from build123d import *

# Parameters (mm, degrees)
SKETCH2_R           = 6
SKETCH2_R_2         = 1.5
BOSS_EXTRUDE1_DEPTH = 1.15
SKETCH3_R           = 4.4
BOSS_EXTRUDE2_DEPTH = 3.2
SKETCH5_R           = 10
SKETCH5_R_2         = 0.75
SKETCH5_R_3         = 1.5
BOSS_EXTRUDE4_DEPTH = 1.15


with BuildPart() as part:
    # Sketch2 → Boss-Extrude1 (new body, symmetric)
    with BuildSketch(Plane(origin=(0, 0, 0), x_dir=(1, 0, 0), z_dir=(0, 1, 0))):
        Circle(SKETCH2_R)
        Circle(SKETCH2_R_2, mode=Mode.SUBTRACT)
    extrude(amount=BOSS_EXTRUDE1_DEPTH, both=True)

    # Sketch3 → Boss-Extrude2 (add)
    with BuildSketch(Plane(origin=(0, 1.15, 0), x_dir=(1, 0, 0), z_dir=(0, 1, 0))):
        Circle(SKETCH3_R)
        with BuildLine():
            Line((0.107421435, 2.898009771), (0.338399731, 2.678709694))
            Line((0.338399731, 2.678709694), (0.61665913, 2.83367809))
            ThreePointArc((0.61665913, 2.83367809), (0.721200673, 2.808891167), (0.824752316, 2.780248841))
            Line((0.824752316, 2.780248841), (0.993936292, 2.510396512))
            Line((0.993936292, 2.510396512), (1.301992734, 2.591295993))
            ThreePointArc((1.301992734, 2.591295993), (1.397085655, 2.541289372), (1.490260976, 2.48779465))
            Line((1.490260976, 2.48779465), (1.587020181, 2.184345885))
            Line((1.587020181, 2.184345885), (1.905517346, 2.186093238))
            ThreePointArc((1.905517346, 2.186093238), (1.985186607, 2.11400902), (2.062131058, 2.039023173))
            Line((2.062131058, 2.039023173), (2.080385755, 1.721044772))
            Line((2.080385755, 1.721044772), (2.389311295, 1.643530205))
            ThreePointArc((2.389311295, 1.643530205), (2.448550984, 1.553897705), (2.504429862, 1.46213237))
            Line((2.504429862, 1.46213237), (2.443033042, 1.149604087))
            Line((2.443033042, 1.149604087), (2.722976028, 0.997698125))
            ThreePointArc((2.722976028, 0.997698125), (2.758063897, 0.896149284), (2.789366126, 0.793370413))
            Line((2.789366126, 0.793370413), (2.652175577, 0.505929549))
            Line((2.652175577, 0.505929549), (2.885546163, 0.289177003))
            ThreePointArc((2.885546163, 0.289177003), (2.894277512, 0.182092507), (2.899036259, 0.074758075))
            Line((2.899036259, 0.074758075), (2.694672167, -0.169534403))
            Line((2.694672167, -0.169534403), (2.866806821, -0.437514174))
            ThreePointArc((2.866806821, -0.437514174), (2.848633027, -0.543405812), (2.826549281, -0.648551587))
            Line((2.826549281, -0.648551587), (2.567852594, -0.834345885))
            Line((2.567852594, -0.834345885), (2.667935462, -1.136714727))
            ThreePointArc((2.667935462, -1.136714727), (2.623998452, -1.234759946), (2.576459817, -1.331110368))
            Line((2.576459817, -1.331110368), (2.279685399, -1.446732346))
            Line((2.279685399, -1.446732346), (2.301427906, -1.764491312))
            ThreePointArc((2.301427906, -1.764491312), (2.234488404, -1.84852957), (2.164481907, -1.930030589))
            Line((2.164481907, -1.930030589), (1.848277186, -1.968215294))
            Line((1.848277186, -1.968215294), (1.790313171, -2.281398419))
            ThreePointArc((1.790313171, -2.281398419), (1.704577232, -2.346149284), (1.616501638, -2.40767989))
            Line((1.616501638, -2.40767989), (1.30073492, -2.366028036))
            Line((1.30073492, -2.366028036), (1.166706475, -2.654956874))
            ThreePointArc((1.166706475, -2.654956874), (1.067561203, -2.696351809), (0.966950626, -2.734045809))
            Line((0.966950626, -2.734045809), (0.671462695, -2.615174535))
            Line((0.671462695, -2.615174535), (0.469791321, -2.861694623))
            ThreePointArc((0.469791321, -2.861694623), (0.363466377, -2.877132634), (0.25664255, -2.888621575))
            Line((0.25664255, -2.888621575), (0, -2.7))
            Line((0, -2.7), (-0.25664255, -2.888621575))
            ThreePointArc((-0.25664255, -2.888621575), (-0.363466377, -2.877132634), (-0.469791321, -2.861694623))
            Line((-0.469791321, -2.861694623), (-0.671462695, -2.615174535))
            Line((-0.671462695, -2.615174535), (-0.966950626, -2.734045809))
            ThreePointArc((-0.966950626, -2.734045809), (-1.067561203, -2.696351809), (-1.166706475, -2.654956874))
            Line((-1.166706475, -2.654956874), (-1.30073492, -2.366028036))
            Line((-1.30073492, -2.366028036), (-1.616501638, -2.40767989))
            ThreePointArc((-1.616501638, -2.40767989), (-1.704577232, -2.346149284), (-1.790313171, -2.281398419))
            Line((-1.790313171, -2.281398419), (-1.848277186, -1.968215294))
            Line((-1.848277186, -1.968215294), (-2.164481907, -1.930030589))
            ThreePointArc((-2.164481907, -1.930030589), (-2.234488404, -1.84852957), (-2.301427906, -1.764491312))
            Line((-2.301427906, -1.764491312), (-2.279685399, -1.446732346))
            Line((-2.279685399, -1.446732346), (-2.576459817, -1.331110368))
            ThreePointArc((-2.576459817, -1.331110368), (-2.623998452, -1.234759946), (-2.667935462, -1.136714727))
            Line((-2.667935462, -1.136714727), (-2.567852594, -0.834345885))
            Line((-2.567852594, -0.834345885), (-2.826549281, -0.648551587))
            ThreePointArc((-2.826549281, -0.648551587), (-2.848633027, -0.543405812), (-2.866806821, -0.437514174))
            Line((-2.866806821, -0.437514174), (-2.694672167, -0.169534403))
            Line((-2.694672167, -0.169534403), (-2.899036259, 0.074758075))
            ThreePointArc((-2.899036259, 0.074758075), (-2.894277512, 0.182092507), (-2.885546163, 0.289177003))
            Line((-2.885546163, 0.289177003), (-2.652175577, 0.505929549))
            Line((-2.652175577, 0.505929549), (-2.789366126, 0.793370413))
            ThreePointArc((-2.789366126, 0.793370413), (-2.758063897, 0.896149284), (-2.722976028, 0.997698125))
            Line((-2.722976028, 0.997698125), (-2.443033042, 1.149604087))
            Line((-2.443033042, 1.149604087), (-2.504429862, 1.46213237))
            ThreePointArc((-2.504429862, 1.46213237), (-2.448550984, 1.553897705), (-2.389311295, 1.643530205))
            Line((-2.389311295, 1.643530205), (-2.080385755, 1.721044772))
            Line((-2.080385755, 1.721044772), (-2.062131058, 2.039023173))
            ThreePointArc((-2.062131058, 2.039023173), (-1.985186607, 2.11400902), (-1.905517346, 2.186093238))
            Line((-1.905517346, 2.186093238), (-1.587020181, 2.184345885))
            Line((-1.587020181, 2.184345885), (-1.490260976, 2.48779465))
            ThreePointArc((-1.490260976, 2.48779465), (-1.397085655, 2.541289372), (-1.301992734, 2.591295993))
            Line((-1.301992734, 2.591295993), (-0.993936292, 2.510396512))
            Line((-0.993936292, 2.510396512), (-0.824752316, 2.780248841))
            ThreePointArc((-0.824752316, 2.780248841), (-0.721200673, 2.808891167), (-0.61665913, 2.83367809))
            Line((-0.61665913, 2.83367809), (-0.338399731, 2.678709694))
            Line((-0.338399731, 2.678709694), (-0.107421435, 2.898009771))
            ThreePointArc((-0.107421435, 2.898009771), (0, 2.9), (0.107421435, 2.898009771))
        make_face(mode=Mode.SUBTRACT)
    extrude(amount=BOSS_EXTRUDE2_DEPTH)

    # Sketch5 → Boss-Extrude4 (add, symmetric)
    with BuildSketch(Plane(origin=(0, 0, 0), x_dir=(1, 0, 0), z_dir=(0, 1, 0))):
        Circle(SKETCH5_R)
        with Locations((0, 7)):
            Circle(SKETCH5_R_2, mode=Mode.SUBTRACT)
        with Locations((-3, 7)):
            Circle(SKETCH5_R_2, mode=Mode.SUBTRACT)
        with Locations((3, 7)):
            Circle(SKETCH5_R_2, mode=Mode.SUBTRACT)
        with Locations((7, 3)):
            Circle(SKETCH5_R_2, mode=Mode.SUBTRACT)
        with Locations((7, 0)):
            Circle(SKETCH5_R_2, mode=Mode.SUBTRACT)
        with Locations((7, -3)):
            Circle(SKETCH5_R_2, mode=Mode.SUBTRACT)
        with Locations((3, -7)):
            Circle(SKETCH5_R_2, mode=Mode.SUBTRACT)
        with Locations((0, -7)):
            Circle(SKETCH5_R_2, mode=Mode.SUBTRACT)
        with Locations((-3, -7)):
            Circle(SKETCH5_R_2, mode=Mode.SUBTRACT)
        with Locations((-7, -3)):
            Circle(SKETCH5_R_2, mode=Mode.SUBTRACT)
        with Locations((-7, 0)):
            Circle(SKETCH5_R_2, mode=Mode.SUBTRACT)
        with Locations((-7, 3)):
            Circle(SKETCH5_R_2, mode=Mode.SUBTRACT)
        Circle(SKETCH5_R_3, mode=Mode.SUBTRACT)
    extrude(amount=BOSS_EXTRUDE4_DEPTH, both=True)


solid = part.part
Geometry: final body of the model. Coordinates: model frame, mm. A direction names the side the tool comes from. Give positions to 0.01 mm unless a question says otherwise; leave off trailing zeros. Order: outer loops, then holes, each group sorted by start corner. A loop starts at its lowest first (then second) coordinate and runs counter-clockwise, first axis right, second up. Notation, with made-up numbers: (48, -38) -> (63, -38) arc R6 cw to (63, -29) -> close; hole circle Ø5 at (89.5, 63). An arc over 180 degrees is marked (long way). Answer as a JSON object with one key per item and string values.
Q1. First-contact query: pin 1 (1.2 mm diameter, centred on x = -3, z = -7, fed in from +Y); pin 2 (1.7 mm diameter, centred on x = -7, z = 0, fed in from +Y); pin 3 (3 mm diameter, centred on y = 2.5, z = 7, fed in from -X); pin 4 (1 mm diameter, centred on x = 7.5, y = -0.5, fed in from +Z). Flat tips, straight axial feed; report the tip coordinate or a pass-through.
Entries:
{"pin 1": "passes through", "pin 2": "stops at y = 1.15", "pin 3": "stops at x = -7.73", "pin 4": "stops at z = 7.14"}
Q2. Section B-B (y = -0.6). State how many separate pieces and enclosed holes the cut face has, plus the area to 3 significant figures.
Entries:
{"separate pieces": "1", "enclosed holes": "13", "area": "286 mm^2"}
Q3. Draft query along Z for faces 1 (the cylindrical face through (-2.17, 0.02, 9.76)), 2 (the cylindrical face through (2.405, -0.016, 7.456)), 3 (the flat face through (0, -1.15, 2)). Return one class per face: released by +Z, released by -Z, zero draft, split by the parting line, or undercut.
Entries:
{"face 1": "split by the parting line", "face 2": "undercut", "face 3": "zero draft"}
Q4. Section D-D (x = -4). Output: boundary loops of the cut face in (y, z).
Entries:
{"outline": "(-1.15, -9.17) -> (1.15, -9.17) -> (1.15, -1.83) -> (4.35, -1.83) -> (4.35, 1.83) -> (1.15, 1.83) -> (1.15, 9.17) -> (-1.15, 9.17) -> close"}
Q5. Material intervals for probe 1 along Z at (x, y) = (0, 0.5); probe 2 along Z at (x, y) = (-7, 0.55); probe 3 along X at (y, z) = (-0.9, -6.75), sorted ascending.
Entries:
{"probe 1": "z = -10 to -7.75, -6.25 to -1.5, 1.5 to 6.25, 7.75 to 10", "probe 2": "z = -7.14 to -3.75, -2.25 to -0.75, 0.75 to 2.25, 3.75 to 7.14", "probe 3": "x = -7.38 to -3.71, -2.29 to -0.71, 0.71 to 2.29, 3.71 to 7.38"}
Q6. Section A-A (z = -7). Output: boundary loops of the cut face in (x, y), plus the area to 3 significant figures.
Entries:
{"outline": "(-7.14, -1.15) -> (-3.75, -1.15) -> (-3.75, 1.15) -> (-7.14, 1.15) -> close; (-2.25, -1.15) -> (-0.75, -1.15) -> (-0.75, 1.15) -> (-2.25, 1.15) -> close; (0.75, -1.15) -> (2.25, -1.15) -> (2.25, 1.15) -> (0.75, 1.15) -> close; (3.75, -1.15) -> (7.14, -1.15) -> (7.14, 1.15) -> (3.75, 1.15) -> close", "area": "22.5 mm^2"}
Q7. Access query for faces 4 (the cylindrical face through (4.197, 2.728, -1.322)), 5 (the cylindrical face through (-3.595, -0.016, 7.456)). Directions: +Z, -Z, +X, -X, +Y, -Y. A direction counts if a zero-diameter tool reaches every point of the face in a straight line with its end or side. Return the directions, or none.
Entries:
{"face 4": "+Y", "face 5": "+Y, -Y"}
Q8. Section C-C (x = -7). Output: boundary loops of the cut face in (y, z).
Entries:
{"outline": "(-1.15, -7.14) -> (1.15, -7.14) -> (1.15, -3.75) -> (-1.15, -3.75) -> close; (-1.15, -2.25) -> (1.15, -2.25) -> (1.15, -0.75) -> (-1.15, -0.75) -> close; (-1.15, 0.75) -> (1.15, 0.75) -> (1.15, 2.25) -> (-1.15, 2.25) -> close; (-1.15, 3.75) -> (1.15, 3.75) -> (1.15, 7.14) -> (-1.15, 7.14) -> close"}
